Here's how the part is built. I have some questions about the finished solid (model axes, mm). A direction names the side the tool comes from. Coordinates: 2 decimals unless noted, no trailing zeros. Write each loop counter-clockwise with the first axis right and the second up, starting at its lowest first coordinate (ties: lowest second). Pieces come first, ordered by that corner, then holes.
Autodesk Inventor part; units mm, degrees
ref_plane "Work Plane1" through (-8.6, -0.4, -2.2) normal (0, 0, 1) x (1, 0, 0)
ref_plane "YZ Plane" through (0, 0, 0) normal (1, 0, 0) x (0, 1, 0)
ref_plane "XZ Plane" through (0, 0, 0) normal (0, 1, 0) x (-1, 0, 0)
sketch "Sketch1" plane through (0, 0, 0) normal (0, 0, 1) x (1, 0, 0)
  line L0 (1, -0.6) -> (1, -5.45)
  line L1 (-15, 0) -> (-11.6, 0)
  line L2 (-6.8, -6.3) -> (-8.6, -6.3)
  line L3 (-8.6, 0) -> (-6.8, 0)
  line L4 (-2.8, 0) -> (-1, 0)
  line L5 (-6.8, -6.3) -> (-8.6, -6.3)
  line L6 (-1, -6.3) -> (-2.8, -6.3)
  line L7 (-8.6, -6.3) -> (-6.8, -6.3)
  line L8 (-6.8, -6.3) -> (-6.8, -6.7)
  line L9 (-6.8, -6.7) -> (-8.6, -6.7)
  line L10 (-8.6, -6.7) -> (-8.6, -6.3)
  line L11 (-8.6, 0) -> (-6.8, 0)
  line L12 (-6.8, 0) -> (-6.8, 0.4)
  line L13 (-6.8, 0.4) -> (-8.6, 0.4)
  line L14 (-8.6, 0.4) -> (-8.6, 0)
  line L15 (-2.8, 0) -> (-1, 0)
  line L16 (-1, 0) -> (-1, 0.4)
  line L17 (-1, 0.4) -> (-2.8, 0.4)
  line L18 (-2.8, 0.4) -> (-2.8, 0)
  line L19 (-2.8, -6.3) -> (-1, -6.3)
  line L20 (-1, -6.3) -> (-1, -6.7)
  line L21 (-1, -6.7) -> (-2.8, -6.7)
  line L22 (-2.8, -6.7) -> (-2.8, -6.3)
  line L23 (-8.6, -5.9) -> (-8.6, -6.3)
  line L24 (-6.8, -5.9) -> (-6.8, -6.3)
  line L25 (-2.8, -5.9) -> (-2.8, -6.3)
  line L26 (-1, -5.9) -> (-1, -6.3)
  line L27 (1, -6.3) -> (-15, -6.3)
  line L28 (-15, -6.3) -> (-15, 0)
  line L29 (-15, 0) -> (1, 0)
  line L30 (1, 0) -> (1, -6.3)
  line L31 (-15, -1.7791) -> (-15, -4.5209)
  point P0 (0, 0)
  dimension "d2" = 0.4
extrude "Extrusion1" add sketch "Sketch1" along normal blind 0.4
sketch "Sketch2" plane through (0, 0, 0) normal (0, 0, -1) x (-1, 0, 0)
  line L0 (8.6, -6.7) -> (6.8, -6.7)
  line L1 (6.8, -6.7) -> (6.8, -6.3)
  line L2 (8.6, -6.7) -> (6.8, -6.7)
  line L3 (6.8, -6.7) -> (6.8, -6.4)
  line L4 (6.8, -6.4) -> (8.6, -6.4)
  line L5 (8.6, -6.4) -> (8.6, -6.7)
  line L6 (2.8, -6.3) -> (2.8, -6.7)
  line L7 (1, -6.7) -> (1, -6.3)
  line L8 (2.8, -6.7) -> (1, -6.7)
  line L9 (1, -6.7) -> (1, -6.4)
  line L10 (1, -6.4) -> (2.8, -6.4)
  line L11 (2.8, -6.4) -> (2.8, -6.7)
  line L12 (1, 0) -> (1, 0.4)
  line L13 (2.8, 0.4) -> (2.8, 0)
  line L14 (1, 0.4) -> (2.8, 0.4)
  line L15 (2.8, 0.4) -> (2.8, 0.1)
  line L16 (2.8, 0.1) -> (1, 0.1)
  line L17 (1, 0.1) -> (1, 0.4)
  line L18 (6.8, 0.4) -> (8.6, 0.4)
  line L19 (8.6, 0.4) -> (8.6, 0)
  line L20 (6.8, 0.4) -> (8.6, 0.4)
  line L21 (8.6, 0.4) -> (8.6, 0.1)
  line L22 (8.6, 0.1) -> (6.8, 0.1)
  line L23 (6.8, 0.1) -> (6.8, 0.4)
  line L24 (6.8, -6.3) -> (2.8, -6.3)
  line L25 (2.8, 0) -> (6.8, 0)
  point P0 (0, 0)
  dimension "d3" = 0.1
  dimension "d4" = 0.1
ref_plane "Work Plane1" through (-8.6, -0.4, -2.2) normal (0, 0, 1) x (1, 0, 0)
extrude "Extrusion2" add sketch "Sketch2" along normal up to surface (2.2 mm away)
sketch "Sketch3" plane through (-8.6, 0.1, 0) normal (0, -1, 0) x (1, 0, 0)
  line L0 (0.1, -1.4) -> (1.7, -1.4)
  line L1 (1.7, -1.4) -> (1.7, -2.2)
  line L2 (1.7, -2.2) -> (0.1, -2.2)
  line L3 (0.1, -2.2) -> (0.1, -1.4)
  line L4 (5.9, -1.4) -> (7.5, -1.4)
  line L5 (7.5, -1.4) -> (7.5, -2.2)
  line L6 (7.5, -2.2) -> (5.9, -2.2)
  line L7 (5.9, -2.2) -> (5.9, -1.4)
  line L8 (1.8, -2.2) -> (1.8, -1.2)
  line L9 (1.8, -1.2) -> (0, -1.2)
  line L10 (0, -2.2) -> (1.8, -2.2)
  line L11 (0, -1.2) -> (0, -2.2)
  line L12 (7.6, -2.2) -> (7.6, -1.2)
  line L13 (5.8, -2.2) -> (7.6, -2.2)
  line L14 (7.6, -1.2) -> (5.8, -1.2)
  line L15 (5.8, -1.2) -> (5.8, -2.2)
  line L16 (1.8, -2.2) -> (0, -2.2)
  line L17 (7.6, -2.2) -> (5.8, -2.2)
  point P0 (8.6, 0)
  point P1 (6.7, -1.2)
  dimension "d7" = 0.1
  dimension "d8" = 0.2
  dimension "d9" = 0.1
  dimension "d10" = 0.1
  dimension "d11" = 0.2
  dimension "d12" = 0.1
extrude "Extrusion3" add sketch "Sketch3" along normal blind 0.35 draft -5 contours L0 L1 L2 L3 | L4 L5 L6 L7
sketch "Sketch4" plane through (-2.8, -6.4, 0) normal (0, 1, 0) x (1, 0, 0)
  line L0 (-4.1, 2.2) -> (-5.7, 2.2)
  line L1 (-5.7, 2.2) -> (-5.7, 1.4)
  line L2 (-4.1, 1.4) -> (-4.1, 2.2)
  line L3 (-5.7, 1.4) -> (-4.1, 1.4)
  line L4 (0.1, 1.4) -> (1.7, 1.4)
  line L5 (0.1, 2.2) -> (0.1, 1.4)
  line L6 (1.7, 2.2) -> (0.1, 2.2)
  line L7 (1.7, 1.4) -> (1.7, 2.2)
  point P0 (2.8, 0)
extrude "Extrusion4" add sketch "Sketch4" along normal blind 0.35 draft -5
chamfer "Chamfer1" distance 0.2 angle 45 4 edges at (-1.9, -0.25, -2.1694) (-7.7, -0.25, -2.1694) (-1.9, -6.05, -2.1694) (-7.7, -6.05, -2.1694)
sketch "Sketch5" plane through (0, 0, 0) normal (0, 0, -1) x (-1, 0, 0)
  line L0 (15, -6.3) -> (11.8, -6.3)
  line L1 (11.8, -6.3) -> (11.8, -5.9)
  line L2 (11.8, -5.9) -> (15, -5.9)
  line L3 (15, -5.9) -> (15, -6.3)
  line L4 (8.6, 0) -> (15, 0)
  line L5 (15, 0) -> (11.8, 0)
  line L6 (11.8, 0) -> (11.8, -0.4)
  line L7 (11.8, -0.4) -> (15, -0.4)
  line L8 (15, -0.4) -> (15, 0)
  line L9 (11.6, 0) -> (11.6, -0.4)
  line L10 (11.6, -5.9) -> (11.6, -6.3)
  point P0 (0, 0)
  dimension "d20" = 0.2
  dimension "d21" = 0.2
extrude "Extrusion5" add sketch "Sketch5" along normal blind 2.4
sketch "Sketch6" plane through (0, 0, 0) normal (0, 0, -1) x (-1, 0, 0)
  line L0 (15, -0.4) -> (15, -5.9)
  line L1 (15, -5.9) -> (14.7, -5.9)
  line L2 (14.7, -5.9) -> (14.7, -0.4)
  line L3 (14.7, -0.4) -> (15, -0.4)
  line L4 (15, -0.4) -> (15, -5.9)
  line L5 (15, -0.4) -> (11.8, -0.4)
  point P0 (0, 0)
  dimension "d24" = 0.3
extrude "Extrusion6" add sketch "Sketch6" along normal blind 2.1
equation "\"d8\" = d11"
equation "\"d9\" = d7"
equation "\"d10\" = d7"
equation "\"d12\" = d7"
equation "\"d21\" = d20"
properties part number "np2_cap_open_top"
1. If I drill on line 1 (Y direction, x = -12.25, z = -0.55); line 2 (Y direction, x = -7, z = -0.95); line 3 (X direction, y = -6.5, z = 0.05), over which ranges is the centre line in solid material (lowest first)?
2. I want a section at A-A (z = -1.05). List the corners of the cut face in (x, y) for me, then the cut area to 3 significant figures.
3. I want a section at B-B (x = -12.75). List the corners of the cut face in (y, z) for me.
4. I want a section at C-C (y = -2.25). List the corners of the cut face in (x, z) for me, then the cut area to 3 significant figures.
5. Thinking about a two-plate mould opening in Y: for faces 4 (the face through (-2, -6.7, -1)), 5 (the face through (-8, 0.4, -1)), 6 (the face through (-13, -0.4, -1)), which applies, pulls with the +Y half, pulls with the -Y half, needs draft (parallel to the pull), parting line crosses it, or undercut?
6. On a 3-axis mill with a long thin cutter (end or side, diameter ignored), from which of +Z, -Z, +X, -X, +Y, -Y can I reach the whole of each face in a straight line? I mean faces 1 (the face through (-13, 0, -1)), 2 (the face through (-14.7, -3, -1)), 3 (the face through (-13, -6.3, -1)). Say none if no direction works.
7. I want a section at D-D (z = 0.25). List the corners of the cut face in (x, y) for me, then the cut area to 3 significant figures.
8. For pin 1 Ø1.2 at (x, z) = (-13, -1.5) entering from -Y; pin 2 Ø1.5 at (y, z) = (-6, -2) entering from +X, each with a flat end and sliding along its axis, tell me the tip position at first contact or that it passes through.
Response values:
1. line 1: y = -6.3 to -5.9, -0.4 to 0
1. line 2: y = -6.7 to -6.4, 0.1 to 0.4
1. line 3: x = -8.6 to -6.8, -2.8 to -1
2. outline: (-15, -6.3) - (-11.8, -6.3) - (-11.8, -5.9) - (-14.7, -5.9) - (-14.7, -0.4) - (-11.8, -0.4) - (-11.8, 0) - (-15, 0) - close; (-8.6, -6.7) - (-6.8, -6.7) - (-6.8, -6.4) - (-8.6, -6.4) - close; (-8.6, 0.1) - (-6.8, 0.1) - (-6.8, 0.4) - (-8.6, 0.4) - close; (-2.8, -6.7) - (-1, -6.7) - (-1, -6.4) - (-2.8, -6.4) - close; (-2.8, 0.1) - (-1, 0.1) - (-1, 0.4) - (-2.8, 0.4) - close
2. area: 6.37 mm2
3. outline: (-6.3, -2.4) - (-5.9, -2.4) - (-5.9, 0) - (-0.4, 0) - (-0.4, -2.4) - (0, -2.4) - (0, 0.4) - (-6.3, 0.4) - close
4. outline: (-15, -2.1) - (-14.7, -2.1) - (-14.7, 0) - (1, 0) - (1, 0.4) - (-15, 0.4) - close
4. area: 7.03 mm2
5. face 4: pulls with the -Y half
5. face 5: pulls with the +Y half
5. face 6: undercut
6. face 1: +Z, -Z, -X, +Y
6. face 2: -Z, +X
6. face 3: +Z, -Z, -X, -Y
7. outline: (-15, -6.3) - (-8.6, -6.3) - (-8.6, -6.7) - (-6.8, -6.7) - (-6.8, -6.3) - (-2.8, -6.3) - (-2.8, -6.7) - (-1, -6.7) - (-1, -6.3) - (1, -6.3) - (1, 0) - (-1, 0) - (-1, 0.4) - (-2.8, 0.4) - (-2.8, 0) - (-6.8, 0) - (-6.8, 0.4) - (-8.6, 0.4) - (-8.6, 0) - (-15, 0) - close
7. area: 104 mm2
8. pin 1: stops at y = -6.3
8. pin 2: stops at x = -1
